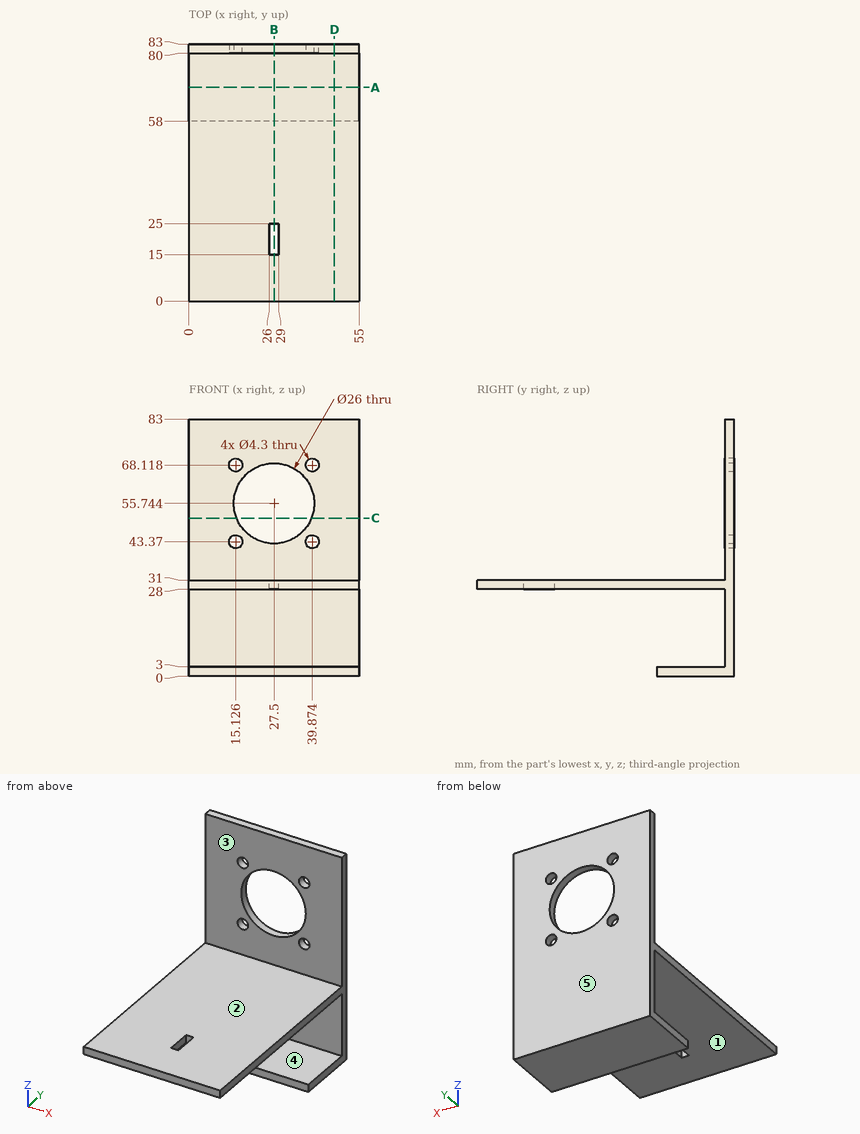
Geometry check sheet. Reference: drawing and pictorial views, mm from the part's lowest x, y, z. A direction names the side the tool comes from. Give positions to 0.01 mm unless a question says otherwise; leave off trailing zeros. Loops run counter-clockwise (first coordinate to the right, second up) from the corner with the lowest first, then second, coordinate; pieces in that order, holes last. Notation, with made-up numbers: (-36, 74) - (0, 74) arc R20 ccw to (0, 95) - close; hole circle Ø3 at (14, 73.5). An arc over 180 degrees is marked (long way). Use CSV: the item, a comma, the result in double quotes. Start each with the question number.
Q1. Section check D-D, the plane x = 47. Record the cut outline in (y, z).
Q2. Scan lines: probe 1 along Z at (x, y) = (27.5, 80.9); probe 2 along Z at (x, y) = (26, 78.5); probe 3 along Y at (x, z) = (48.5, 10). Record each from-to range of solid material in increasing order. Write a range as from..to.
Q3. Section check B-B, the plane x = 27.5. Record the cut outline in (y, z).
Q4. Access from +Z, -Z, +X, -X, +Y, -Y to the whole of each face (thin tool, end or side, straight path). Record for the marked faces 4 and 5.
Q5. Go/stop test with flat-tipped pins: pin 1 Ø10 at (x, y) = (20, 21.5) entering from +Z; pin 2 Ø5 at (x, z) = (15.13, 43.37) entering from -Y; pin 3 Ø23.5 at (x, z) = (27.5, 55.74) entering from -Y; pin 4 Ø3.5 at (x, z) = (21, 1.5) entering from -Y. Record where each tip stops, or that it passes through.
Q6. Release check for a two-part mould opening along Z. For the marked faces 1, 2 and 3 record: +Z half, -Z half, draft (parallel to the pull), parting line (faces both ways), or undercut.
Q7. Section check A-A, the plane y = 69. Record the cut outline in (x, z), and give its area (3 significant figures).
Q8. Section check C-C, the plane z = 51. Record the cut outline in (x, y).
Findings below:
1,outline,"(0, 28) - (80, 28) - (80, 3) - (58, 3) - (58, 0) - (83, 0) - (83, 83) - (80, 83) - (80, 31) - (0, 31) - close"
2,probe 1,"z = 0..42.74, 68.74..83"
2,probe 2,"z = 0..3, 28..31"
2,probe 3,"y = 80..83"
3,outline,"(0, 28) - (15, 28) - (15, 31) - (0, 31) - close; (25, 28) - (80, 28) - (80, 3) - (58, 3) - (58, 0) - (83, 0) - (83, 42.74) - (80, 42.74) - (80, 31) - (25, 31) - close; (80, 68.74) - (83, 68.74) - (83, 83) - (80, 83) - close"
4,face 4,"+X, -X, -Y"
4,face 5,"+Z, -Z, +X, -X, +Y"
5,pin 1,"stops at z = 31"
5,pin 2,"stops at y = 80"
5,pin 3,"passes through"
5,pin 4,"stops at y = 58"
6,face 1,"undercut"
6,face 2,"+Z half"
6,face 3,"draft"
7,outline,"(0, 0) - (55, 0) - (55, 3) - (0, 3) - close; (0, 28) - (55, 28) - (55, 31) - (0, 31) - close"
7,area,"330 mm^2"
8,outline,"(0, 80) - (15.4, 80) - (15.4, 83) - (0, 83) - close; (39.6, 80) - (55, 80) - (55, 83) - (39.6, 83) - close"
